For this review, take the finished solid that the model builds, in its own axes (mm). Face numbers are marked on the shaded views. Give positions to 0.01 mm unless a question says otherwise; leave off trailing zeros. Order: outer loops, then holes, each group sorted by start corner. A loop starts at its lowest first (then second) coordinate and runs counter-clockwise, first axis right, second up. Notation, with made-up numbers: (-2, 44) -> (16, 44) arc R24 cw to (16, 62) -> close; hole circle Ø10 at (-3, 63). An arc over 180 degrees is marked (long way). Return JSON: item names as keys, results as strings. Group by question number.
1) Add section C-C (z = -20). Give the boundary of the cut face in (x, y).
2) To check wall thickness, follow line 1 along Y through (x, z) = (9.5, -55); line 2 along Z through (x, y) = (8.75, 32); line 3 along Z through (x, y) = (4.75, 32). State the ranges of each line that lie inside material, in increasing order.
3) Insertion check: P1, Ø1.5, axis at x = 12.5, z = -112, coming from the -Y side; P2, Ø3.5, axis at x = 12.5, z = -127.5, coming from the +Y side; P3, Ø4, axis at y = 55, z = -115.5, coming from the +X side; P4, Ø5, axis at x = 7.5, y = 69, coming from the -Z side. Each pin has a flat end and moves straight along its axis. Give the tip position at first contact, or say it passes through.
4) Add section A-A (z = -120). Give the boundary of the cut face in (x, y).
5) The part is to be moulded in two halves that separate along Z. For the marked faces 1 and 2, say which applies: released by +Z, released by -Z, zero draft, split by the parting line, or undercut.
6) Add section B-B (y = 60). Give the boundary of the cut face in (x, z), then the cut area to 3 significant figures.
7) Add section D-D (y = 44.9). Give the boundary of the cut face in (x, z).
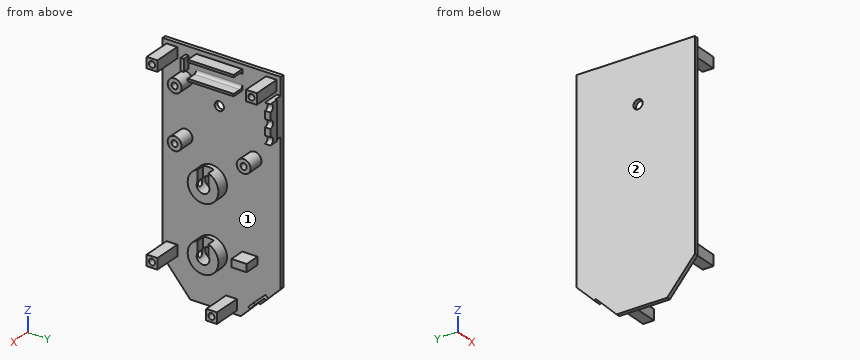
from build123d import *

# Parameters (mm, degrees)
BASE_DEPTH               = 2.5
SKETCH2_R                = 4.5
SKETCH2_R_2              = 2
SKETCH2_W                = 5
SKETCH2_H                = 10
PCB_MOUNT_DEPTH          = 10.2
BOSS_EXTRUDE14_REACH     = 178.254
BOSS_EXTRUDE14_START     = -4.5
SKETCH24_R               = 2
SKETCH3_R                = 10
SKETCH3_R_2              = 4.15
BOSS_EXTRUDE3_DEPTH      = 8
SKETCH4_W                = 7.770089688
SKETCH4_H                = 7
CUT_EXTRUDE1_DEPTH       = 5
SKETCH5_R                = 2
CUT_EXTRUDE2_DEPTH       = 160.985280573
SKETCH13_W               = 11
SKETCH13_H               = 25
BOSS_EXTRUDE8_DEPTH      = 2.5
BOSS_EXTRUDE9_DEPTH      = 1
BOSS_EXTRUDE9_DEPTH_BACK = 2.5
SKETCH15_W               = 6
SKETCH15_H               = 25
CUT_EXTRUDE4_REACH       = 174.265
SKETCH16_R               = 2.5
BOSS_EXTRUDE5_START      = -2.5
BOSS_EXTRUDE5_DEPTH      = 2.5
BOSS_EXTRUDE6_DEPTH      = 2.5
BOSS_EXTRUDE7_DEPTH      = 1.3
SKETCH19_W               = 1.5
SKETCH19_H               = 30
BOSS_EXTRUDE11_DEPTH     = 8
FILLET1_R                = 2
SKETCH20_W               = 8
SKETCH20_H               = 2
BOSS_EXTRUDE12_DEPTH     = 4.5
SKETCH21_W               = 7
SKETCH21_H               = 7
BOSS_EXTRUDE13_DEPTH     = 18.5
SKETCH22_R               = 2
CUT_EXTRUDE5_DEPTH       = 4.5
CUT_EXTRUDE6_REACH       = 175.014
SKETCH25_R               = 3


with BuildPart() as part:
    # Sketch1 → Base (new body)
    with BuildSketch(Plane(origin=(0, 0, 0), x_dir=(0, 0, -1), z_dir=(1, 0, 0))):
        Polygon((0, 0), (0, 77), (127, 77), (153, 51), (153, 18), (132, 0), align=None)
    extrude(amount=BASE_DEPTH)

    # Sketch2 → PCB_Mount (add)
    # profile 1 of 4: a face of its own
    with BuildSketch(Plane(origin=(2.5, 0, 0), x_dir=(0, 0, -1), z_dir=(1, 0, 0))):
        with Locations(Location((20, 15, 0), (0, 0, 180))):
            Circle(SKETCH2_R)
        with Locations((20, 15)):
            Circle(SKETCH2_R_2, mode=Mode.SUBTRACT)
    # profile 2 of 4: a face of its own
    with BuildSketch(Plane(origin=(2.5, 0, 0), x_dir=(0, 0, -1), z_dir=(1, 0, 0))):
        with Locations(Location((55, 15, 0), (0, 0, 180))):
            Circle(SKETCH2_R)
        with Locations((55, 15)):
            Circle(SKETCH2_R_2, mode=Mode.SUBTRACT)
    # profile 3 of 4: a face of its own
    with BuildSketch(Plane(origin=(2.5, 0, 0), x_dir=(0, 0, -1), z_dir=(1, 0, 0))):
        with Locations(Location((55, 60, 0), (0, 0, 180))):
            Circle(SKETCH2_R)
        with Locations((55, 60)):
            Circle(SKETCH2_R_2, mode=Mode.SUBTRACT)
    # profile 4 of 4: a face of its own
    with BuildSketch(Plane(origin=(2.5, 0, 0), x_dir=(0, 0, -1), z_dir=(1, 0, 0))):
        with Locations((116, 57)):
            Rectangle(SKETCH2_W, SKETCH2_H)
    extrude(amount=PCB_MOUNT_DEPTH)

    # Sketch24 → Boss-Extrude14 (add, up to next)
    with BuildSketch(Plane(origin=(12.7, 0, 0), x_dir=(0, 0, -1), z_dir=(1, 0, 0)).offset(BOSS_EXTRUDE14_START), mode=Mode.PRIVATE) as boss_extrude14_sk1:
        with Locations((55, 60)):
            Circle(SKETCH24_R)
    boss_extrude14_tool1 = extrude(boss_extrude14_sk1.sketch, amount=-BOSS_EXTRUDE14_REACH, mode=Mode.PRIVATE) - part.part
    # Sketch24 → Boss-Extrude14 (add, up to next)
    with BuildSketch(Plane(origin=(12.7, 0, 0), x_dir=(0, 0, -1), z_dir=(1, 0, 0)).offset(BOSS_EXTRUDE14_START), mode=Mode.PRIVATE) as boss_extrude14_sk2:
        with Locations((55, 15)):
            Circle(SKETCH24_R)
    boss_extrude14_tool2 = extrude(boss_extrude14_sk2.sketch, amount=-BOSS_EXTRUDE14_REACH, mode=Mode.PRIVATE) - part.part
    # Sketch24 → Boss-Extrude14 (add, up to next)
    with BuildSketch(Plane(origin=(12.7, 0, 0), x_dir=(0, 0, -1), z_dir=(1, 0, 0)).offset(BOSS_EXTRUDE14_START), mode=Mode.PRIVATE) as boss_extrude14_sk3:
        with Locations((20, 15)):
            Circle(SKETCH24_R)
    boss_extrude14_tool3 = extrude(boss_extrude14_sk3.sketch, amount=-BOSS_EXTRUDE14_REACH, mode=Mode.PRIVATE) - part.part
    add(boss_extrude14_tool1.solids().sort_by_distance((8.2, 60, -55))[0])
    add(boss_extrude14_tool2.solids().sort_by_distance((8.2, 15, -55))[0])
    add(boss_extrude14_tool3.solids().sort_by_distance((8.2, 15, -20))[0])

    # Sketch3 → Boss-Extrude3 (add)
    # profile 1 of 2: a face of its own
    with BuildSketch(Plane(origin=(2.5, 0, 0), x_dir=(0, 0, -1), z_dir=(1, 0, 0))):
        with Locations(Location((77, 32, 0), (0, 0, 180))):
            Circle(SKETCH3_R)
        with Locations((77, 32)):
            Circle(SKETCH3_R_2, mode=Mode.SUBTRACT)
    # profile 2 of 2: a face of its own
    with BuildSketch(Plane(origin=(2.5, 0, 0), x_dir=(0, 0, -1), z_dir=(1, 0, 0))):
        with Locations(Location((120, 32, 0), (0, 0, 180))):
            Circle(SKETCH3_R)
        with Locations((120, 32)):
            Circle(SKETCH3_R_2, mode=Mode.SUBTRACT)
    extrude(amount=BOSS_EXTRUDE3_DEPTH)

    # Sketch4 → Cut-Extrude1 (cut)
    with BuildSketch(Plane(origin=(10.5, 0, 0), x_dir=(0, 0, -1), z_dir=(1, 0, 0))):
        with Locations((70.885044844, 32)):
            Rectangle(SKETCH4_W, SKETCH4_H)
        with Locations((113.885044844, 32)):
            Rectangle(SKETCH4_W, SKETCH4_H)
    extrude(amount=-CUT_EXTRUDE1_DEPTH, mode=Mode.SUBTRACT)

    # Sketch5 → Cut-Extrude2 (cut, through all)
    with BuildSketch(Plane(origin=(0, 32, 0), x_dir=(1, 0, 0), z_dir=(0, 1, 0))):
        with Locations(Location((7.5, 77, 0), (0, 0, 270))):
            Circle(SKETCH5_R)
        with Locations(Location((7.5, 120, 0), (0, 0, 270))):
            Circle(SKETCH5_R)
    extrude(amount=-CUT_EXTRUDE2_DEPTH, mode=Mode.SUBTRACT)

    # Sketch13 → Boss-Extrude8 (add)
    with BuildSketch(Plane(origin=(0, 77, 0), x_dir=(1, 0, 0), z_dir=(0, 1, 0))):
        with Locations((8, 24)):
            Rectangle(SKETCH13_W, SKETCH13_H)
    extrude(amount=-BOSS_EXTRUDE8_DEPTH)

    # Sketch15 → Boss-Extrude9 (add, two sides: drawn at the far end of the back side and taken through both)
    with BuildSketch(Plane(origin=(0, 77, 0), x_dir=(1, 0, 0), z_dir=(0, 1, 0)).offset(-BOSS_EXTRUDE9_DEPTH_BACK)):
        with Locations((10.5, 24)):
            Rectangle(SKETCH15_W, SKETCH15_H)
    extrude(amount=BOSS_EXTRUDE9_DEPTH + BOSS_EXTRUDE9_DEPTH_BACK)

    # Sketch16 → Cut-Extrude4 (cut, up to next)
    with BuildSketch(Plane(origin=(0, 78, 0), x_dir=(1, 0, 0), z_dir=(0, 1, 0)), mode=Mode.PRIVATE) as cut_extrude4_sk1:
        with Locations((13.5, 24)):
            Circle(SKETCH16_R)
    cut_extrude4_tool1 = extrude(cut_extrude4_sk1.sketch, amount=-CUT_EXTRUDE4_REACH, mode=Mode.PRIVATE) & part.part
    # Sketch16 → Cut-Extrude4 (cut, up to next)
    with BuildSketch(Plane(origin=(0, 78, 0), x_dir=(1, 0, 0), z_dir=(0, 1, 0)), mode=Mode.PRIVATE) as cut_extrude4_sk2:
        with Locations((13.5, 34)):
            Circle(SKETCH16_R)
    cut_extrude4_tool2 = extrude(cut_extrude4_sk2.sketch, amount=-CUT_EXTRUDE4_REACH, mode=Mode.PRIVATE) & part.part
    # Sketch16 → Cut-Extrude4 (cut, up to next)
    with BuildSketch(Plane(origin=(0, 78, 0), x_dir=(1, 0, 0), z_dir=(0, 1, 0)), mode=Mode.PRIVATE) as cut_extrude4_sk3:
        with Locations((13.5, 14)):
            Circle(SKETCH16_R)
    cut_extrude4_tool3 = extrude(cut_extrude4_sk3.sketch, amount=-CUT_EXTRUDE4_REACH, mode=Mode.PRIVATE) & part.part
    add(cut_extrude4_tool1.solids().sort_by_distance((13.5, 78, -24))[0], mode=Mode.SUBTRACT)
    add(cut_extrude4_tool2.solids().sort_by_distance((13.5, 78, -34))[0], mode=Mode.SUBTRACT)
    add(cut_extrude4_tool3.solids().sort_by_distance((13.5, 78, -14))[0], mode=Mode.SUBTRACT)

    # Sketch9 → Boss-Extrude5 (add)
    with BuildSketch(Plane.ZY.offset(BOSS_EXTRUDE5_START)):
        Polygon((-127, 77), (-128.697056275, 77), (-140.364318164, 65.33273811), (-139.515790027, 64.484209973), align=None)
    extrude(amount=BOSS_EXTRUDE5_DEPTH)

    # Sketch10 → Boss-Extrude6 (add)
    with BuildSketch(Plane(origin=(2.5, 0, 0), x_dir=(0, 0, -1), z_dir=(1, 0, 0))):
        Polygon((140.364318164, 65.33273811), (136.828784258, 68.868272016), (135.061017306, 67.100505063), (138.596551211, 63.564971157), align=None)
    extrude(amount=BOSS_EXTRUDE6_DEPTH)

    # Sketch12 → Boss-Extrude7 (add)
    with BuildSketch(Plane(origin=(0, 101.080761184, -101.080761184), x_dir=(1, 0, 0), z_dir=(0, -0.7071067811865475, 0.7071067811865477))):
        with BuildLine():
            Line((5, -48.055339059), (5, -53.055339059))
            Line((5, -53.055339059), (13.5, -53.055339059))
            ThreePointArc((13.5, -53.055339059), (11, -50.555339059), (13.5, -48.055339059))
            Line((13.5, -48.055339059), (5, -48.055339059))
        make_face()
    extrude(amount=-BOSS_EXTRUDE7_DEPTH)

    # Sketch19 → Boss-Extrude11 (add)
    with BuildSketch(Plane(origin=(2.5, 0, 0), x_dir=(0, 0, -1), z_dir=(1, 0, 0))):
        with Locations((3.75, 37)):
            Rectangle(SKETCH19_W, SKETCH19_H)
        with Locations((15.25, 37)):
            Rectangle(SKETCH19_W, SKETCH19_H)
    extrude(amount=BOSS_EXTRUDE11_DEPTH)

    # Fillet1
    fillet1_edges = [part.edges().sort_by_distance(p)[0] for p in [
        (2.5, 37, -4.5),
        (2.5, 37, -14.5),
    ]]
    fillet(fillet1_edges, radius=FILLET1_R)

    # Sketch20 → Boss-Extrude12 (add)
    with BuildSketch(Plane(origin=(2.5, 0, 0), x_dir=(0, 0, -1), z_dir=(1, 0, 0))):
        with Locations((9.5, 16)):
            Rectangle(SKETCH20_W, SKETCH20_H)
    extrude(amount=BOSS_EXTRUDE12_DEPTH)

    # Sketch21 → Boss-Extrude13 (add)
    with BuildSketch(Plane(origin=(2.5, 0, 0), x_dir=(0, 0, -1), z_dir=(1, 0, 0))):
        with Locations((6.1, 70.9)):
            Rectangle(SKETCH21_W, SKETCH21_H)
        with Locations((6.1, 6.1)):
            Rectangle(SKETCH21_W, SKETCH21_H)
        with Locations((125.9, 6.1)):
            Rectangle(SKETCH21_W, SKETCH21_H)
        with Locations((146.9, 44.9)):
            Rectangle(SKETCH21_W, SKETCH21_H)
    extrude(amount=BOSS_EXTRUDE13_DEPTH)

    # Sketch22 → Cut-Extrude5 (cut)
    with BuildSketch(Plane(origin=(21, 0, 0), x_dir=(0, 0, -1), z_dir=(1, 0, 0))):
        with Locations((6.1, 6.1)):
            Circle(SKETCH22_R)
        with Locations((6.1, 70.9)):
            Circle(SKETCH22_R)
        with Locations((146.9, 44.9)):
            Circle(SKETCH22_R)
        with Locations((125.9, 6.1)):
            Circle(SKETCH22_R)
    extrude(amount=-CUT_EXTRUDE5_DEPTH, mode=Mode.SUBTRACT)

    # Sketch25 → Cut-Extrude6 (cut, up to next)
    with BuildSketch(Plane.ZY, mode=Mode.PRIVATE) as cut_extrude6_sk1:
        with Locations((-30, 37)):
            Circle(SKETCH25_R)
    cut_extrude6_tool1 = extrude(cut_extrude6_sk1.sketch, amount=-CUT_EXTRUDE6_REACH, mode=Mode.PRIVATE) & part.part
    add(cut_extrude6_tool1.solids().sort_by_distance((0, 37, -30))[0], mode=Mode.SUBTRACT)


solid = part.part
Evaluation:
{
 "1": {"outline": "(0, 0) -> (2.5, 0) -> (2.5, 10.5) -> (12.7, 10.5) -> (12.7, 13) -> (8.2, 13) -> (8.2, 17) -> (12.7, 17) -> (12.7, 19.5) -> (2.5, 19.5) -> (2.5, 74.5) -> (13.5, 74.5) -> (13.5, 78) -> (7.5, 78) -> (7.5, 77) -> (0, 77) -> close"},
 "2": {"line 1": "10.5 to 13, 17 to 19.5, 55.5 to 58, 62 to 64.5", "line 2": "-130 to -124.15, -87 to -81.15, -16 to -14.5, -4.5 to -3", "line 3": "-130 to -124.15, -115.85 to -110, -87 to -81.15, -72.85 to -67, -16 to -14.5, -4.5 to -3"},
 "3": {"P1": "through", "P2": "y = 9.6", "P3": "x = 12.7", "P4": "z = -137.5"},
 "4": {"outline": "(0, 0) -> (2.5, 0) -> (2.5, 22) -> (5.5, 22) -> (5.5, 27.85) -> (2.5, 27.85) -> (2.5, 36.15) -> (10.5, 36.15) -> (10.5, 42) -> (2.5, 42) -> (2.5, 77) -> (0, 77) -> close; (9.5, 22) -> (10.5, 22) -> (10.5, 27.85) -> (9.5, 27.85) -> close"},
 "5": {"face 1": "undercut", "face 2": "zero draft"},
 "6": {"outline": "(0, -144) -> (2.5, -144) -> (2.5, -118.5) -> (12.7, -118.5) -> (12.7, -113.5) -> (2.5, -113.5) -> (2.5, -59.5) -> (12.7, -59.5) -> (12.7, -57) -> (8.2, -57) -> (8.2, -53) -> (12.7, -53) -> (12.7, -50.5) -> (2.5, -50.5) -> (2.5, 0) -> (0, 0) -> close", "area": "485 mm^2"},
 "7": {"outline": "(0, -153) -> (2.5, -153) -> (2.5, -150.4) -> (21, -150.4) -> (21, -148.9) -> (16.5, -148.9) -> (16.5, -144.9) -> (21, -144.9) -> (21, -143.4) -> (2.5, -143.4) -> (2.5, -16) -> (10.5, -16) -> (10.5, -14.5) -> (4.5, -14.5) arc R2 cw to (2.5, -12.5) -> (2.5, -6.5) arc R2 cw to (4.5, -4.5) -> (10.5, -4.5) -> (10.5, -3) -> (2.5, -3) -> (2.5, 0) -> (0, 0) -> close"}
}
